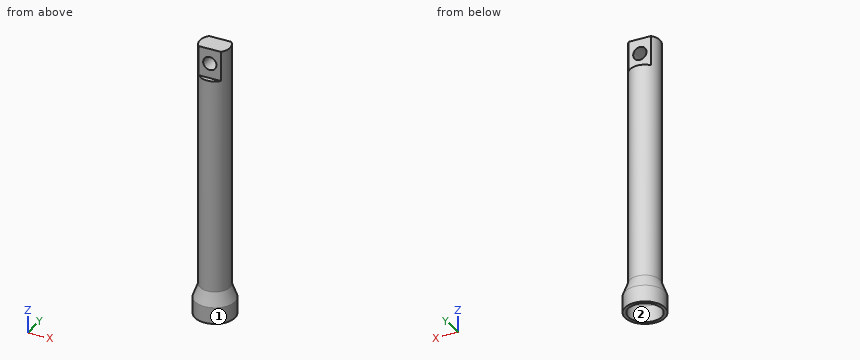
from build123d import *

# Parameters (mm, degrees)
SKETCH3_R               = 22.5
SKETCH3_R_2             = 17.5
BOSS_EXTRUDE1_DEPTH     = 320
SKETCH4_R               = 22.5
BOSS_EXTRUDE2_DEPTH     = 50
SKETCH5_W               = 33.541019662
SKETCH5_H               = 20
CUT_EXTRUDE1_DEPTH      = 45
SKETCH6_R               = 10
CUT_EXTRUDE3_DEPTH      = 16
CUT_EXTRUDE3_DEPTH_BACK = 46


with BuildPart() as part:
    # Sketch2 → Revolve1 (revolve)
    with BuildSketch(Plane(origin=(0, 0, 0), x_dir=(1, 0, 0), z_dir=(0, 1, 0))):
        Polygon((-30, 0), (-30, -25), (-22.5, -45), (-17.5, -45), (-25, -25), (-25, 0), align=None)
    revolve(axis=Axis((0, 0, 47.25), (0, 0, -1)))

    # Sketch3 → Boss-Extrude1 (add)
    with BuildSketch(Plane.XY.offset(45)):
        Circle(SKETCH3_R)
        Circle(SKETCH3_R_2, mode=Mode.SUBTRACT)
    extrude(amount=BOSS_EXTRUDE1_DEPTH)

    # Sketch4 → Boss-Extrude2 (add)
    with BuildSketch(Plane.XY.offset(365)):
        Circle(SKETCH4_R)
    extrude(amount=BOSS_EXTRUDE2_DEPTH)

    # Sketch5 → Cut-Extrude1 (cut)
    with BuildSketch(Plane.XY.offset(415)):
        with Locations((0, 25)):
            Rectangle(SKETCH5_W, SKETCH5_H)
        with Locations((0, -25)):
            Rectangle(SKETCH5_W, SKETCH5_H)
    extrude(amount=-CUT_EXTRUDE1_DEPTH, mode=Mode.SUBTRACT)

    # Sketch6 → Cut-Extrude3 (cut, two sides)
    with BuildSketch(Plane(origin=(0, 15, 0), x_dir=(1, 0, 0), z_dir=(0, 1, 0))) as cut_extrude3_sk:
        with Locations((0, -392.5)):
            Circle(SKETCH6_R)
    extrude(amount=CUT_EXTRUDE3_DEPTH, mode=Mode.SUBTRACT)
    extrude(cut_extrude3_sk.sketch, amount=-CUT_EXTRUDE3_DEPTH_BACK, mode=Mode.SUBTRACT)


solid = part.part
Geometry check sheet. Reference: the model listing, model coordinates, mm. Face numbers are marked on the shaded views. Round coordinates to 2 decimals unless told otherwise and drop trailing zeros. Loops run counter-clockwise (first coordinate to the right, second up) from the corner with the lowest first, then second, coordinate; pieces in that order, holes last. Notation, with made-up numbers: (65, 23) - (89, 23) arc R27 ccw to (89, 62) - close; hole circle Ø2 at (-23.5, 11.5). An arc over 180 degrees is marked (long way). Answer as CSV lines item,"result".
(1) Cross-section at A-A, the plane x = 0. Enter the section's corners in (y, z), and give its area (4 significant figures).
Output values:
outline,"(-30, 0) - (-25, 0) - (-25, 25) - (-17.5, 45) - (-17.5, 365) - (17.5, 365) - (17.5, 45) - (25, 25) - (25, 0) - (30, 0) - (30, 25) - (22.5, 45) - (22.5, 370) - (15, 370) - (15, 382.5) - (-15, 382.5) - (-15, 370) - (-22.5, 370) - (-22.5, 45) - (-30, 25) - close; (-15, 402.5) - (15, 402.5) - (15, 415) - (-15, 415) - close"
area,"4,625 mm²"
(2) Release check for a two-part mould opening along Y. For the marked faces 1 and 2 record: released by +Y, released by -Y, zero draft, split by the parting line, or undercut.
Output values:
face 1,"split by the parting line"
face 2,"undercut"
(3) Material ranges on line 1 along X through (y, z) = (0, 215.5); line 2 along Z through (x, y) = (0, 5.75); line 3 along Y through (x, z) = (-1, 293.5), recorded low to high.
Output values:
line 1,"x = -22.5 to -17.5, 17.5 to 22.5"
line 2,"z = 365 to 382.5, 402.5 to 415"
line 3,"y = -22.48 to -17.47, 17.47 to 22.48"
(4) Cross-section at B-B, the plane z = 392.5. Enter the section's corners in (x, y).
Output values:
outline,"(-16.77, -15) - (-10, -15) - (-10, 15) - (-16.77, 15) arc R22.5 ccw to start; (10, -15) - (16.77, -15) arc R22.5 ccw to (16.77, 15) - (10, 15) - close"
(5) Cross-section at C-C, the plane y = 0. Enter the section's corners in (x, z), and give its area (3 significant figures).
Output values:
outline,"(-30, 0) - (-25, 0) - (-25, 25) - (-17.5, 45) - (-17.5, 365) - (17.5, 365) - (17.5, 45) - (25, 25) - (25, 0) - (30, 0) - (30, 25) - (22.5, 45) - (22.5, 415) - (-22.5, 415) - (-22.5, 45) - (-30, 25) - close; hole circle Ø20 at (0, 392.5)"
area,"5,590 mm²"
(6) Depth check by flat-ended pin: pin 1 Ø5 at (y, z) = (16, 279.5) entering from -X; pin 2 Ø8 at (x, z) = (21.5, 357) entering from +Y; pin 3 Ø5 at (x, z) = (11.5, 186) entering from -Y. Enter the tip coordinate at first touch or a pass-through.
Output values:
pin 1,"stops at x = -18"
pin 2,"stops at y = 14.14"
pin 3,"stops at y = -20.62"
(7) Cross-section at D-D, the plane z = 66.5. Enter the section's corners in (x, y), and give its area (3 significant figures).
Output values:
outline,"circle Ø45 at (0, 0); hole circle Ø35 at (0, 0)"
area,"628 mm²"
